Here's how the part is built. I have some questions about the finished solid (model axes, mm). Coordinates: 2 decimals unless noted, no trailing zeros. Write each loop counter-clockwise with the first axis right and the second up, starting at its lowest first coordinate (ties: lowest second). Pieces come first, ordered by that corner, then holes.
Item 1: Please list where these lines run through material, in increasing order: line 1 (Y direction, x = -91.5, z = 1.8); line 2 (Y direction, x = -18, z = 1.8); line 3 (Y direction, x = -32.5, z = 0.15).
Item 2: I want a section at A-A (x = -129.5). Please give me the cut outline in (y, z), and give its area (3 significant figures).
Item 3: I want a section at B-B (z = 1.3). Count the separate pieces of the cut face and the enclosed holes in it, and give its area (3 significant figures).
Item 4: I'm going to push flat-ended pins straight in: P1, Ø0.8, axis at y = 2, z = 1.5, coming from the +X side; P2, Ø1.3, axis at x = -28.5, z = 1.5, coming from the -Y side; P3, Ø0.8, axis at x = -20.5, z = 1, coming from the +Y side. Where does each tip first touch, or does it pass through?
Item 5: I want a section at C-C (y = -130). Please give me the cut outline in (x, z).
from build123d import *

# Parameters (mm, degrees)
SKETCH2_R           = 2.3495
SKETCH2_R_2         = 2.0955
BOSS_EXTRUDE1_DEPTH = 2.54
SKETCH3_W           = 31.75
SKETCH3_H           = 44.323
BOSS_EXTRUDE2_DEPTH = 2.54
SKETCH4_R           = 2.413
CUT_EXTRUDE1_DEPTH  = 238.743265275
SKETCH5_R           = 2.413
CUT_EXTRUDE2_DEPTH  = 238.743265275
SKETCH6_R           = 2.413
CUT_EXTRUDE3_DEPTH  = 238.743265275
SKETCH7_R           = 2.413
CUT_EXTRUDE4_DEPTH  = 238.743265275
SKETCH8_W           = 7.994763
SKETCH8_H           = 21.113506736
SKETCH8_W_2         = 21.493659396
SKETCH8_H_2         = 28.960940125
CUT_EXTRUDE5_DEPTH  = 238.743265275


with BuildPart() as part:
    # Sketch2 → Boss-Extrude1 (new body)
    with BuildSketch(Plane(origin=(0, 0, 0), x_dir=(-1, 0, 0), z_dir=(0, 0, 1))):
        Polygon((-2.930050059, 168.708281075), (38.709428475, 168.708281075), (38.709428475, 189.536281075), (143.497061781, 189.536281075), (104.617436481, 110.859781075), (72.867436481, 110.859781075), (72.867436481, 66.536781075), (104.617436481, 66.536781075), (143.497061781, -12.139718925), (38.709428475, -12.139718925), (38.709428475, 8.688281075), (-2.930050059, 8.688281075), align=None)
        with Locations(Location((41.95655448, 160.961281075, 0), (0, 0, 180))):
            Circle(SKETCH2_R, mode=Mode.SUBTRACT)
        with Locations(Location((90.673911143, 180.011281075, 0), (0, 0, 180))):
            Circle(SKETCH2_R, mode=Mode.SUBTRACT)
        with Locations(Location((90.673911143, -2.614718925, 0), (0, 0, 180))):
            Circle(SKETCH2_R, mode=Mode.SUBTRACT)
        with Locations(Location((3.035061781, 117.209781075, 0), (0, 0, 180))):
            Circle(SKETCH2_R, mode=Mode.SUBTRACT)
        with Locations(Location((3.035061781, 60.186781075, 0), (0, 0, 180))):
            Circle(SKETCH2_R, mode=Mode.SUBTRACT)
        with Locations(Location((41.95655448, 16.435281075, 0), (0, 0, 180))):
            Circle(SKETCH2_R_2, mode=Mode.SUBTRACT)
    extrude(amount=BOSS_EXTRUDE1_DEPTH)

    # Sketch3 → Boss-Extrude2 (add)
    with BuildSketch(Plane.XY.offset(2.54)):
        with Locations((-88.742436481, -88.698281075)):
            Rectangle(SKETCH3_W, SKETCH3_H)
    extrude(amount=-BOSS_EXTRUDE2_DEPTH)

    # Sketch4 → Cut-Extrude1 (cut, through all)
    with BuildSketch(Plane.XY.offset(2.54)):
        with Locations((-94.457436481, -69.711781075)):
            Circle(SKETCH4_R)
        with Locations((-83.027436481, -69.711781075)):
            Circle(SKETCH4_R)
        with Locations((-28.311949941, -69.711781075)):
            Circle(SKETCH4_R)
        with Locations((-9.261949941, -69.711781075)):
            Circle(SKETCH4_R)
        with Locations(Location((-9.261949941, -107.684781075, 0), (0, 0, 180))):
            Circle(SKETCH4_R)
        with Locations(Location((-28.311949941, -107.684781075, 0), (0, 0, 180))):
            Circle(SKETCH4_R)
        with Locations(Location((-83.027436481, -107.684781075, 0), (0, 0, 180))):
            Circle(SKETCH4_R)
        with Locations(Location((-94.457436481, -107.684781075, 0), (0, 0, 180))):
            Circle(SKETCH4_R)
    extrude(amount=-CUT_EXTRUDE1_DEPTH, mode=Mode.SUBTRACT)

    # Sketch5 → Cut-Extrude2 (cut, through all)
    with BuildSketch(Plane.XY.offset(2.54)):
        with Locations((-31.738991634, -58.273080522)):
            Circle(SKETCH5_R)
    extrude(amount=-CUT_EXTRUDE2_DEPTH, mode=Mode.SUBTRACT)

    # Sketch6 → Cut-Extrude3 (cut, through all)
    with BuildSketch(Plane.XY.offset(2.54)):
        with Locations((-32.511395831, -23.991781075)):
            Circle(SKETCH6_R)
    extrude(amount=-CUT_EXTRUDE3_DEPTH, mode=Mode.SUBTRACT)

    # Sketch7 → Cut-Extrude4 (cut, through all)
    with BuildSketch(Plane.XY.offset(2.54)):
        with Locations((-32.140467993, -155.071444629)):
            Circle(SKETCH7_R)
        with Locations((-32.140467993, -120.781444629)):
            Circle(SKETCH7_R)
    extrude(amount=-CUT_EXTRUDE4_DEPTH, mode=Mode.SUBTRACT)

    # Sketch8 → Cut-Extrude5 (cut, through all)
    with BuildSketch(Plane.XY.offset(2.54)):
        with Locations((-36.236046975, 1.868472293)):
            Rectangle(SKETCH8_W, SKETCH8_H)
        with Locations((-29.486598777, -183.188751137)):
            Rectangle(SKETCH8_W_2, SKETCH8_H_2)
    extrude(amount=-CUT_EXTRUDE5_DEPTH, mode=Mode.SUBTRACT)


solid = part.part
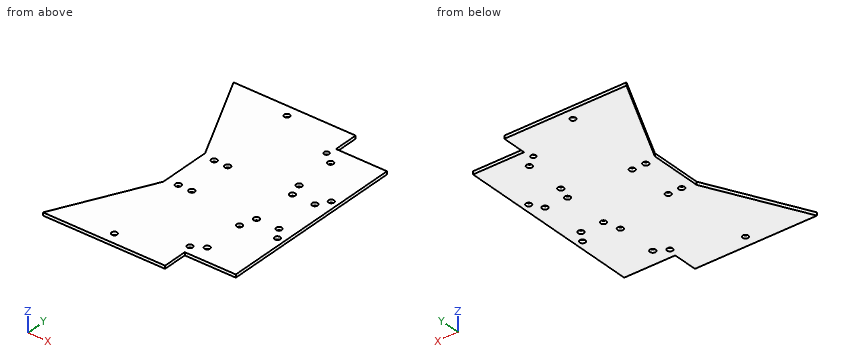
Answer:
1. line 1: y = -189.54 to -182.21, -177.81 to 0.42, 4.81 to 12.14
1. line 2: y = -168.71 to -8.69
1. line 3: y = -168.71 to -157.46, -152.69 to -123.17, -118.4 to -60.56, -55.98 to -26.4, -21.58 to -8.69
2. outline: (-189.54, 0) - (-161.21, 0) - (-161.21, 2.54) - (-189.54, 2.54) - close; (-16.18, 0) - (12.14, 0) - (12.14, 2.54) - (-16.18, 2.54) - close
2. area: 144 mm2
3. separate pieces: 1
3. enclosed holes: 18
3. area: 22,600 mm2
4. P1: stops at x = -40.23
4. P2: stops at y = -168.71
4. P3: stops at y = -8.69
5. outline: (-114.08, 0) - (2.93, 0) - (2.93, 2.54) - (-114.08, 2.54) - close
